The model under review builds one solid part; all positions refer to its coordinate system, in mm. A direction names the side the tool comes from. Round coordinates to 2 decimals unless told otherwise and drop trailing zeros. Loops run counter-clockwise (first coordinate to the right, second up) from the corner with the lowest first, then second, coordinate; pieces in that order, holes last. Notation, with made-up numbers: (19, -12.5) -> (60, -12.5) arc R11 ccw to (60, -5.5) -> close; hole circle Ø9 at (-24, 85.5). An arc over 180 degrees is marked (long way). Write each question's results on one line, items separated by ' | '. Start each with the question number.
Item 1: We need section D-D (x = 0). Give the boundary of the cut face in (y, z).
Item 2: We need section B-B (z = 27). Give the boundary of the cut face in (x, y), and give its area (3 significant figures).
Item 3: Mouldability with a two-part tool opening along Z and no side actions: class faces 4 (the flat face through (15, 10, 18)), 5 (the cylindrical face through (14.816, -2.168, 29.048)) as pulls with the +Z half, pulls with the -Z half, needs draft (parallel to the pull), parting line crosses it, or undercut.
Item 4: We need section C-C (z = 31). Give the boundary of the cut face in (x, y), and give its area (3 significant figures).
Item 5: Tool access review of faces 1 (the flat face through (-15, 10, 18)), 2 (the flat face through (0, -12.512, 18)), 3 (the flat face through (21, -3, 18)): name each direction out of +Z, -Z, +X, -X, +Y, -Y from which nothing blocks a thin tool from reaching the whole face with its end or side.
Item 6: We need section A-A (y = 0). Give the boundary of the cut face in (x, z), and give its area (3 significant figures).
Item 7: Clearance check with flat-ended pins moving along their axes: pin 1 Ø5.5 at (x, z) = (3, 25) entering from -Y; pin 2 Ø3 at (y, z) = (8, 25) entering from +X; pin 3 Ø10 at (x, z) = (-15.5, 18) entering from +Y; pin 4 Ø4 at (x, z) = (-16.5, 7.5) entering from +Y. State where each tip first meets the part, or that it passes through.
Item 8: For L1, parallel to Z at x = 15.25, y = 1.5; L2, parallel to X at y = -0.25, z = 16.5; L3, parallel to X at y = 3.25, z = 32.5, list the stretches that pass through material, from the lowest coordinate up. Write a range as from..to.
from build123d import *

# Parameters (mm, degrees)
SKETCH1_R           = 6
BOSS_EXTRUDE1_DEPTH = 36
CUT_EXTRUDE1_REACH  = 30
SKETCH2_R           = 2


with BuildPart() as part:
    # Sketch1 → Boss-Extrude1 (new body)
    with BuildSketch(Plane.XY):
        Polygon((-7.376347734, 14), (-10.704853009, 10), (-19.287228785, 10), (-21, 7.941693254), (-21, -14), (-12.193167268, -14), (-10.704853009, -14), (-9.216538749, -12.511685741), (9.216538749, -12.511685741), (10.704853009, -14), (12.193167268, -14), (21, -14), (21, 7.941693254), (19.287228785, 10), (10.704853009, 10), (7.376347734, 14), align=None)
        Circle(SKETCH1_R, mode=Mode.SUBTRACT)
    extrude(amount=BOSS_EXTRUDE1_DEPTH)

    # Sketch2 → Cut-Extrude1 (cut, up to next)
    with BuildSketch(Plane.XZ.offset(14), mode=Mode.PRIVATE) as cut_extrude1_sk1:
        with Locations((-15.25, 31)):
            Circle(SKETCH2_R)
    cut_extrude1_tool1 = extrude(cut_extrude1_sk1.sketch, amount=-CUT_EXTRUDE1_REACH, mode=Mode.PRIVATE) & part.part
    add(cut_extrude1_tool1.solids().sort_by_distance((-15.25, -14, 31))[0], mode=Mode.SUBTRACT)
    # Sketch2 → Cut-Extrude1 (cut, up to next)
    with BuildSketch(Plane.XZ.offset(14), mode=Mode.PRIVATE) as cut_extrude1_sk2:
        with Locations((15.25, 31)):
            Circle(SKETCH2_R)
    cut_extrude1_tool2 = extrude(cut_extrude1_sk2.sketch, amount=-CUT_EXTRUDE1_REACH, mode=Mode.PRIVATE) & part.part
    add(cut_extrude1_tool2.solids().sort_by_distance((15.25, -14, 31))[0], mode=Mode.SUBTRACT)
    # Sketch2 → Cut-Extrude1 (cut, up to next)
    with BuildSketch(Plane.XZ.offset(14), mode=Mode.PRIVATE) as cut_extrude1_sk3:
        with Locations((15.25, 5)):
            Circle(SKETCH2_R)
    cut_extrude1_tool3 = extrude(cut_extrude1_sk3.sketch, amount=-CUT_EXTRUDE1_REACH, mode=Mode.PRIVATE) & part.part
    add(cut_extrude1_tool3.solids().sort_by_distance((15.25, -14, 5))[0], mode=Mode.SUBTRACT)
    # Sketch2 → Cut-Extrude1 (cut, up to next)
    with BuildSketch(Plane.XZ.offset(14), mode=Mode.PRIVATE) as cut_extrude1_sk4:
        with Locations((-15.25, 5)):
            Circle(SKETCH2_R)
    cut_extrude1_tool4 = extrude(cut_extrude1_sk4.sketch, amount=-CUT_EXTRUDE1_REACH, mode=Mode.PRIVATE) & part.part
    add(cut_extrude1_tool4.solids().sort_by_distance((-15.25, -14, 5))[0], mode=Mode.SUBTRACT)


solid = part.part
Here are the results:
1) outline: (-12.51, 0) -> (-6, 0) -> (-6, 36) -> (-12.51, 36) -> close; (6, 0) -> (14, 0) -> (14, 36) -> (6, 36) -> close
2) outline: (-21, -14) -> (-10.7, -14) -> (-9.22, -12.51) -> (9.22, -12.51) -> (10.7, -14) -> (21, -14) -> (21, 7.94) -> (19.29, 10) -> (10.7, 10) -> (7.38, 14) -> (-7.38, 14) -> (-10.7, 10) -> (-19.29, 10) -> (-21, 7.94) -> close; hole circle Ø12 at (0, 0) | area: 934 mm2
3) face 4: needs draft | face 5: undercut
4) outline: (-21, -14) -> (-17.25, -14) -> (-17.25, 10) -> (-19.29, 10) -> (-21, 7.94) -> close; (-13.25, -14) -> (-10.7, -14) -> (-9.22, -12.51) -> (9.22, -12.51) -> (10.7, -14) -> (13.25, -14) -> (13.25, 10) -> (10.7, 10) -> (7.38, 14) -> (-7.38, 14) -> (-10.7, 10) -> (-13.25, 10) -> close; (17.25, -14) -> (21, -14) -> (21, 7.94) -> (19.29, 10) -> (17.25, 10) -> close; hole circle Ø12 at (0, 0) | area: 742 mm2
5) face 1: +Z, -Z, -X, +Y | face 2: +Z, -Z, -Y | face 3: +Z, -Z, +X, +Y, -Y
6) outline: (-21, 0) -> (-6, 0) -> (-6, 36) -> (-21, 36) -> close; (6, 0) -> (21, 0) -> (21, 36) -> (6, 36) -> close; hole circle Ø4 at (-15.25, 5); hole circle Ø4 at (-15.25, 31); hole circle Ø4 at (15.25, 5); hole circle Ø4 at (15.25, 31) | area: 1,030 mm2
7) pin 1: stops at y = -12.51 | pin 2: stops at x = 21 | pin 3: stops at y = 10.25 | pin 4: stops at y = 10
8) L1: z = 0..3, 7..29, 33..36 | L2: x = -21..-5.99, 5.99..21 | L3: x = -21..-16.57, -13.93..-5.04, 5.04..13.93, 16.57..21
